```python
from build123d import *

# Parameters (mm, degrees)
F0_W     = 356
F0_H     = 246
F1_DEPTH = 2
F2_W     = 10
F2_H     = 236
F3_DEPTH = 5


with BuildPart() as f1:
    # F0 (on Top) → F1 (new body)
    with BuildSketch(Plane.XY):
        Rectangle(F0_W, F0_H)
    extrude(amount=F1_DEPTH)

    # F2 (on Top) → F3 (cut)
    with BuildSketch(Plane.XY):
        with Locations((-164.875, 0)):
            Rectangle(F2_W, F2_H)
        with Locations((-149.875, 0)):
            Rectangle(F2_W, F2_H)
        with Locations((-134.875, 0)):
            Rectangle(F2_W, F2_H)
        with Locations((-119.875, 0)):
            Rectangle(F2_W, F2_H)
        with Locations((-104.875, 0)):
            Rectangle(F2_W, F2_H)
        with Locations((-89.875, 0)):
            Rectangle(F2_W, F2_H)
        with Locations((-74.875, 0)):
            Rectangle(F2_W, F2_H)
        with Locations((-59.875, 0)):
            Rectangle(F2_W, F2_H)
        with Locations((-44.875, 0)):
            Rectangle(F2_W, F2_H)
        with Locations((-29.875, 0)):
            Rectangle(F2_W, F2_H)
        with Locations((-14.875, 0)):
            Rectangle(F2_W, F2_H)
        with Locations((0.125, 0)):
            Rectangle(F2_W, F2_H)
        with Locations((15.125, 0)):
            Rectangle(F2_W, F2_H)
        with Locations((30.125, 0)):
            Rectangle(F2_W, F2_H)
        with Locations((45.125, 0)):
            Rectangle(F2_W, F2_H)
        with Locations((60.125, 0)):
            Rectangle(F2_W, F2_H)
        with Locations((75.125, 0)):
            Rectangle(F2_W, F2_H)
        with Locations((90.125, 0)):
            Rectangle(F2_W, F2_H)
        with Locations((105.125, 0)):
            Rectangle(F2_W, F2_H)
        with Locations((120.125, 0)):
            Rectangle(F2_W, F2_H)
        with Locations((135.125, 0)):
            Rectangle(F2_W, F2_H)
        with Locations((150.125, 0)):
            Rectangle(F2_W, F2_H)
        with Locations((165.125, 0)):
            Rectangle(F2_W, F2_H)
    extrude(amount=F3_DEPTH, mode=Mode.SUBTRACT)


solid = f1.part
```
Build history of the part. All positions in model axes, mm. Round coordinates to 2 decimals unless told otherwise and drop trailing zeros. Loops run counter-clockwise (first coordinate to the right, second up) from the corner with the lowest first, then second, coordinate; pieces in that order, holes last.
Item 1: Saw through at A-A (x = 121). List the corners of the cut face in (y, z).
Item 2: Pin check, flat tip, straight feed: P1, Ø4, axis at x = 103, y = 87.5, coming from the +Z side. Stop position of the tip, or through.
Item 3: Drill centre line: line 1 along Y through (x, z) = (116, 0.15). Where is it in solid material? Low to high.
Item 4: Saw through at B-B (y = 12). State how many separate pieces and enclosed holes the cut face has, then the cut area to 3 significant figures.
Worked answers:
1. outline: (-123, 0) - (-118, 0) - (-118, 2) - (-123, 2) - close; (118, 0) - (123, 0) - (123, 2) - (118, 2) - close
2. P1: passes through
3. line 1: y = -123 to -118, 118 to 123
4. separate pieces: 24
4. enclosed holes: 0
4. area: 252 mm2
